Check sheet for the modelled part. Datum: model origin and axes. Units: mm. Face numbers are marked on the shaded views. Round coordinates to 2 decimals unless told otherwise and drop trailing zeros. Loops run counter-clockwise (first coordinate to the right, second up) from the corner with the lowest first, then second, coordinate; pieces in that order, holes last. Notation, with made-up numbers: (-4, -16) - (16, -16) arc R15 cw to (16, -8) - close; hole circle Ø2 at (21, 29.25). An arc over 180 degrees is marked (long way). Return JSON: item names as keys, results as strings.
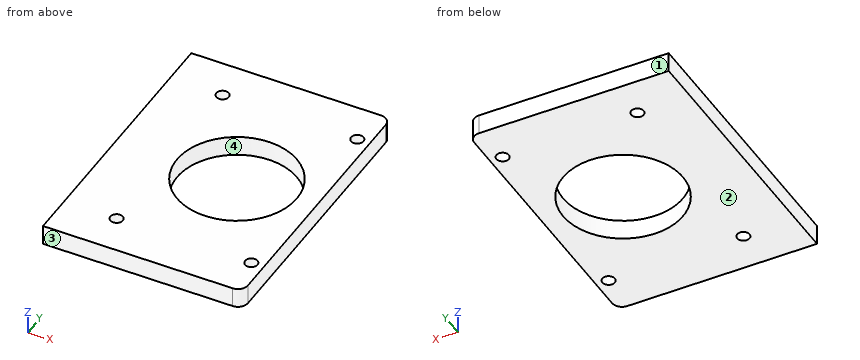
Autodesk Inventor part; units mm, degrees
ref_plane "YZ Plane" through (0, 0, 0) normal (1, 0, 0) x (0, 1, 0)
ref_plane "XZ Plane" through (0, 0, 0) normal (0, 1, 0) x (-1, 0, 0)
ref_plane "XY Plane" through (0, 0, 0) normal (0, 0, 1) x (1, 0, 0)
sketch "Sketch1" plane through (0, 0, 0) normal (0, 0, 1) x (1, 0, 0)
  line L0 (-3.175, 0) -> (-63.5, 0)
  line L1 (0, 3.175) -> (0, 85.725)
  line L2 (-3.175, 88.9) -> (-63.5, 88.9)
  line L3 (-63.5, 88.9) -> (-63.5, 0)
  circle A0 centre (-3.9688, 76.2) radius 1.9844
  circle A1 centre (-3.9688, 12.7) radius 1.9844
  circle A2 centre (-46.8313, 12.7) radius 1.9812
  circle A3 centre (-46.8313, 76.2) radius 1.9812
  arc A4 (0, 85.725) -> (-3.175, 88.9) centre (-3.175, 85.725) ccw
  arc A5 (-3.175, 0) -> (0, 3.175) centre (-3.175, 3.175) ccw
  point P0 (0, 0)
  point P1 (0, 88.9)
  dimension "d0" = 63.5
  dimension "d1" = 88.9
  dimension "d2" = 3.9688
  dimension "d3" = 3.9688
  dimension "d4" = 3.9624
  dimension "d5" = 3.9624
  dimension "d6" = 12.7
  dimension "d7" = 12.7
  dimension "d8" = 12.7
  dimension "d9" = 3.9688
  dimension "d10" = 3.9688
  dimension "d11" = 16.6687
  dimension "d12" = 12.7
  dimension "d13" = 16.6687
  dimension "d19" = 3.175
extrude "Plate1" add sketch "Sketch1" along normal blind 6.35
sketch "Sketch2" plane through (0, 0, 6.35) normal (0, 0, 1) x (1, 0, 0)
  line L0 (0, 85.725) -> (0, 3.175)
  line L1 (-63.5, 88.9) -> (-3.175, 88.9)
  line L2 (0, 44.45) -> (-25.4, 44.45)
  circle A0 centre (-25.4, 44.45) radius 19.05
  point P0 (0, 0)
  point P1 (0, 88.9)
  dimension "d15" = 25.4
  dimension "d16" = 38.1
extrude "Cut1" cut sketch "Sketch2" against normal blind 6.35
equation "\"d17\" = Thickness"
equation "\"BendRadius\" = Thickness"
equation "\"BendReliefWidth\" = Thickness"
equation "\"BendReliefDepth\" = 0.5 * Thickness"
equation "\"CornerReliefSize\" = 4 * Thickness"
equation "\"MinimumRemnant\" = 2 * Thickness"
equation "\"TransitionRadius\" = BendRadius"
equation "\"JacobiRadiusSize\" = BendRadius"
equation "\"GapSize\" = Thickness"
equation "\"d14\" = BendRadius"
properties part number "bearing faceplate"
Q1. Draft check along Y on the marked faces 1, 2, 3 and 4. Enter one of: released by +Y, released by -Y, zero draft, split by the parting line, or undercut.
Answer key:
{"face 1": "released by +Y", "face 2": "zero draft", "face 3": "released by -Y", "face 4": "undercut"}
Q2. Sectioned sample at D-D (z = 5). Enter the section's corners in (x, y) (3 decimals), plus the area to 3 significant figures.
Answer key:
{"outline": "(-63.5, 0) - (-3.175, 0) arc R3.175 ccw to (0, 3.175) - (0, 85.725) arc R3.175 ccw to (-3.175, 88.9) - (-63.5, 88.9) - close; hole circle Ø3.962 at (-46.831, 12.7); hole circle Ø3.962 at (-46.831, 76.2); hole circle Ø38.1 at (-25.4, 44.45); hole circle Ø3.969 at (-3.969, 12.7); hole circle Ø3.969 at (-3.969, 76.2)", "area": "4,450 mm²"}
Q3. Scan lines: probe 1 along Y at (x, z) = (-47, 5); probe 2 along Y at (x, z) = (-3.5, 4.5); probe 3 along Y at (x, z) = (-25.4, 4.5). Record each from-to range of solid material in increasing order. Write a range as [from, to].
Answer key:
{"probe 1": "y = [0, 10.73], [14.67, 74.23], [78.17, 88.9]", "probe 2": "y = [0, 10.77], [14.63, 74.27], [78.13, 88.9]", "probe 3": "y = [0, 25.4], [63.5, 88.9]"}
Q4. Sectioned sample at B-B (x = -25.4). Enter the section's corners in (y, z).
Answer key:
{"outline": "(0, 0) - (25.4, 0) - (25.4, 6.35) - (0, 6.35) - close; (63.5, 0) - (88.9, 0) - (88.9, 6.35) - (63.5, 6.35) - close"}
Q5. Depth check by flat-ended pin: P1, Ø1, axis at y = 44, z = 2.5, coming from the +X side; P2, Ø23, axis at x = -25.4, y = 44.45, coming from the -Z side. Enter the tip coordinate at first touch or a pass-through.
Answer key:
{"P1": "stops at x = 0", "P2": "passes through"}
Q6. Sectioned sample at C-C (y = 44.45). Enter the section's corners in (x, z), plus the area to 3 significant figures.
Answer key:
{"outline": "(-63.5, 0) - (-44.45, 0) - (-44.45, 6.35) - (-63.5, 6.35) - close; (-6.35, 0) - (0, 0) - (0, 6.35) - (-6.35, 6.35) - close", "area": "161 mm²"}
Q7. Sectioned sample at A-A (y = 12.7). Enter the section's corners in (x, z), plus the area to 3 significant figures.
Answer key:
{"outline": "(-63.5, 0) - (-48.81, 0) - (-48.81, 6.35) - (-63.5, 6.35) - close; (-44.85, 0) - (-5.95, 0) - (-5.95, 6.35) - (-44.85, 6.35) - close; (-1.98, 0) - (0, 0) - (0, 6.35) - (-1.98, 6.35) - close", "area": "353 mm²"}
